Answer from the drawing. Dimensions are ordinates in mm from the lowest x, y and z of the part. Give positions to 0.01 mm unless a question says otherwise; leave off trailing zeros. Write each loop counter-clockwise with the first axis right and the second up, starting at its lowest first coordinate (ties: lowest second). Pieces come first, ordered by that corner, then holes. Notation, with made-up numbers: M -4,77 L 33,77 A16 ccw 33,83 Z; hole C -2,20.5 d5. An arc over 180 degrees is marked long. Answer as a JSON object with one key per item and string values.
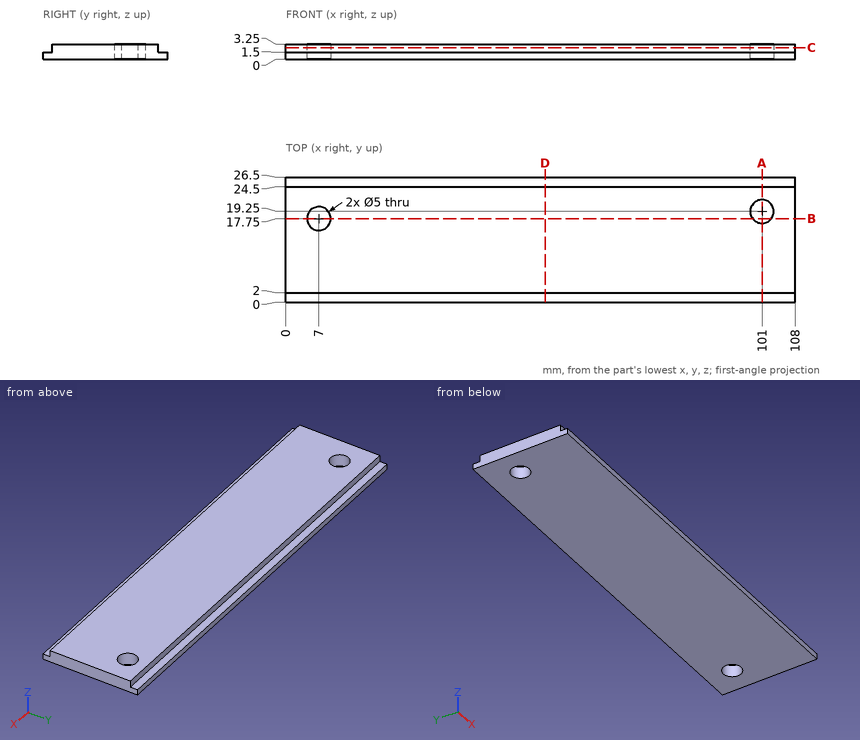
1. Consider line 1 along Y through (x, z) = (101, 1.9); line 2 along Y through (x, z) = (7, 1.75); line 3 along Z through (x, y) = (97, 1.75). Determine where each line is inside the solid, lowest interval first.
Verdict:
{"line 1": "y = 2 to 16.75, 21.75 to 24.5", "line 2": "y = 2 to 15.25, 20.25 to 24.5", "line 3": "z = 0 to 1.5"}
2. A cutting plane is placed at D-D, the plane x = 55. Give the vertices of the cut face in (y, z), plus the area to 3 significant figures.
Verdict:
{"outline": "M 0,0 L 26.5,0 L 26.5,1.5 L 24.5,1.5 L 24.5,3.25 L 2,3.25 L 2,1.5 L 0,1.5 Z", "area": "79.1 mm2"}
3. Flat-ended cylindrical pins translate along their axes: pin 1 (1.5 mm diameter, centred on x = 50, z = 2.5, fed in from -Y); pin 2 (1.6 mm diameter, centred on x = 28.5, y = 1, fed in from +Z). Find the tip coordinate at first contact, or state that the pin passes through.
Verdict:
{"pin 1": "stops at y = 2", "pin 2": "stops at z = 1.5"}
4. A cutting plane is placed at B-B, the plane y = 17.75. Give the vertices of the cut face in (x, z).
Verdict:
{"outline": "M 0,0 L 4.5,0 L 4.5,3.25 L 0,3.25 Z; M 9.5,0 L 99,0 L 99,3.25 L 9.5,3.25 Z; M 103,0 L 108,0 L 108,3.25 L 103,3.25 Z"}
5. A cutting plane is placed at C-C, the plane z = 2.5. Give the vertices of the cut face in (x, y).
Verdict:
{"outline": "M 0,2 L 108,2 L 108,24.5 L 0,24.5 Z; hole C 7,17.75 d5; hole C 101,19.25 d5"}
6. A cutting plane is placed at A-A, the plane x = 101. Give the vertices of the cut face in (y, z).
Verdict:
{"outline": "M 0,0 L 16.75,0 L 16.75,3.25 L 2,3.25 L 2,1.5 L 0,1.5 Z; M 21.75,0 L 26.5,0 L 26.5,1.5 L 24.5,1.5 L 24.5,3.25 L 21.75,3.25 Z"}
